CAD build for the part. Positions are in the model's coordinates, mm. Give positions to 0.01 mm unless a question says otherwise; leave off trailing zeros. Write each loop counter-clockwise with the first axis right and the second up, starting at its lowest first coordinate (ties: lowest second). Pieces come first, ordered by that corner, then holes. Notation, with made-up numbers: (44, 29) - (66, 29) arc R22 ccw to (66, 54) - close; hole circle Ø11 at (-17, 64). An arc over 180 degrees is marked (long way). Answer as a JSON object with one key per item and string values.
Autodesk Inventor part; units mm, degrees
ref_plane "YZ Plane" through (0, 0, 0) normal (1, 0, 0) x (0, 1, 0)
ref_plane "XZ Plane" through (0, 0, 0) normal (0, 1, 0) x (-1, 0, 0)
ref_plane "XY Plane" through (0, 0, 0) normal (0, 0, 1) x (1, 0, 0)
sketch "Sketch1" plane through (0, 0, 0) normal (0, 0, 1) x (1, 0, 0)
  line L0 (-47.2309, 58.7326) -> (-58.3434, 58.7326)
  line L1 (-69.4559, 84.1326) -> (-69.4559, 69.8451)
  arc A0 (-69.4559, 69.8451) -> (-58.3434, 58.7326) centre (-58.3434, 69.8451) ccw
  line L2 (-69.4559, 69.8451) -> (-69.4559, 86.6091)
  line L3 (-47.2309, 96.8326) -> (-58.3434, 96.8326)
  line L4 (-69.4559, 85.7201) -> (-69.4559, 86.6091)
  arc A1 (-58.3434, 96.8326) -> (-69.4559, 85.7201) centre (-58.3434, 85.7201) ccw
  line L5 (-47.2309, 46.0326) -> (-66.2809, 46.0326)
  line L6 (-98.0309, 77.7826) -> (-98.0309, 77.7826)
  line L7 (-66.2809, 109.5326) -> (-47.2309, 109.5326)
  arc A2 (-66.2809, 109.5326) -> (-98.0309, 77.7826) centre (-66.2809, 77.7826) ccw
  arc A3 (-98.0309, 77.7826) -> (-66.2809, 46.0326) centre (-66.2809, 77.7826) ccw
  circle A4 centre (-47.2309, 103.1826) radius 2.0955
  circle A5 centre (-47.2309, 52.3826) radius 2.0955
  circle A6 centre (-85.3309, 93.5778) radius 2.0828
  circle A7 centre (-85.3309, 61.9874) radius 2.0828
  line L8 (-47.2309, 96.8326) -> (-21.8309, 96.8326)
  line L9 (-15.4809, 103.1826) -> (-15.4809, 103.1826)
  line L10 (-21.8309, 109.5326) -> (-47.2309, 109.5326)
  line L11 (-47.2309, 58.7326) -> (-21.8309, 58.7326)
  line L12 (-15.4809, 52.3826) -> (-15.4809, 52.3826)
  line L13 (-21.8309, 46.0326) -> (-47.2309, 46.0326)
  arc A8 (-15.4809, 52.3826) -> (-21.8309, 58.7326) centre (-21.8309, 52.3826) ccw
  arc A9 (-21.8309, 46.0326) -> (-15.4809, 52.3826) centre (-21.8309, 52.3826) ccw
  arc A10 (-21.8309, 96.8326) -> (-15.4809, 103.1826) centre (-21.8309, 103.1826) ccw
  arc A11 (-15.4809, 103.1826) -> (-21.8309, 109.5326) centre (-21.8309, 103.1826) ccw
  line L14 (-75.7109, 63.3494) -> (-75.7109, 92.2158)
  arc A12 (-76.923, 92.8904) -> (-76.923, 62.6748) centre (-67.5536, 77.7826) ccw
  arc A13 (-75.7109, 92.2158) -> (-76.923, 92.8904) centre (-76.5047, 92.2158) ccw
  arc A14 (-76.923, 62.6748) -> (-75.7109, 63.3494) centre (-76.5047, 63.3494) ccw
  point P0 (-69.4559, 58.7326)
  point P1 (-15.4809, 58.7326)
  point P2 (-75.7109, 93.5778)
  point P3 (-75.7109, 61.9874)
  dimension "d11" = 22.225
  dimension "d12" = 11.1125
  dimension "d13" = 11.1125
  dimension "d14" = 31.75
  dimension "d15" = 31.75
  dimension "d16" = 4.191
  dimension "d17" = 4.191
  dimension "d18" = 4.1656
  dimension "d19" = 4.1656
  dimension "d21" = 6.35
  dimension "d27" = 0.7937
extrude "Extrusion1" add sketch "Sketch1" along normal blind 1.5875 contours L11 A8 A9 L13 L5 A3 A2 L7 L10 A11 A10 L8 L3 A1 L2 L1 A0 L0 | A14 A12 A13 L14
sketch "Sketch2" plane through (-21.8309, 46.0326, 1.5875) normal (0, 0, 1) x (1, 0, 0)
  circle A0 centre (-24.7079, -19.05) radius 2.3114
  arc A1 (-31.0579, -19.05) -> (-18.4424, -20.0828) centre (-24.7079, -19.05) ccw
  line L0 (-31.0579, -19.05) -> (-31.0579, -6.35)
  line L1 (-44.45, 0) -> (0, 0)
  arc A2 (-31.0579, -6.35) -> (-37.4079, 0) centre (-37.4079, -6.35) ccw
  arc A3 (0, 0) -> (0, 12.7) centre (0, 6.35) ccw
  arc A4 (1.2054, 0.1155) -> (-18.4424, -20.0828) centre (5.886, -24.0929) ccw
  circle A5 centre (25.4, 6.35) radius 2.0955
  line L2 (0, 63.5) -> (-44.45, 63.5)
  arc A6 (0, 50.8) -> (0, 63.5) centre (0, 57.15) ccw
  arc A7 (25.4, 0) -> (25.4, 12.7) centre (25.4, 6.35) ccw
  line L3 (0, 12.7) -> (25.4, 12.7)
  line L4 (0, 0) -> (25.4, 0)
  circle A8 centre (25.4, 57.15) radius 2.0955
  arc A9 (25.4, 50.8) -> (25.4, 63.5) centre (25.4, 57.15) ccw
  line L5 (25.4, 50.8) -> (0, 50.8)
  line L6 (0, 63.5) -> (25.4, 63.5)
  arc A10 (0, 50.8) -> (0, 63.5) centre (0, 57.15) ccw
  point P0 (21.8309, -46.0326)
  point P1 (-31.0579, 0)
  point P2 (0.6434, 0)
  dimension "d22" = 4.6228
  dimension "d24" = 6.35
  dimension "d29" = 4.191
  dimension "d31" = 4.191
  dimension "d32" = 12.7
extrude "Extrusion2" add sketch "Sketch2" against normal blind 1.5875
sketch "Sketch5" plane through (3.5691, 103.1826, 0) normal (0, 0, -1) x (-1, 0, 0)
  line L0 (0, 6.35) -> (69.85, 6.35)
  line L1 (12.7, 0) -> (20.6375, 0) construction
  arc A0 (69.85, -57.15) -> (69.85, 6.35) centre (69.85, -25.4) ccw
  line L2 (69.85, 6.35) -> (50.8, 6.35)
  line L3 (0, 6.35) -> (0, 6.35)
  circle A1 centre (15.875, 25.4) radius 1.905
  arc A2 (0, 6.35) -> (0, -6.35) centre (0, 0) ccw
  line L4 (-6.35, 0) -> (-6.35, 26.9875)
  circle A3 centre (0, 25.4) radius 1.905
  line L5 (-3.175, 30.1625) -> (15.875, 30.1625)
  line L6 (20.6375, 19.05) -> (20.6375, 26.9875)
  line L7 (17.4625, 30.1625) -> (15.875, 30.1625)
  arc A4 (20.6375, 26.9875) -> (17.4625, 30.1625) centre (17.4625, 26.9875) ccw
  arc A5 (-3.175, 30.1625) -> (-6.35, 26.9875) centre (-3.175, 26.9875) ccw
  line L8 (33.3375, 6.35) -> (50.8, 6.35)
  arc A6 (20.6375, 19.05) -> (33.3375, 6.35) centre (33.3375, 19.05) ccw
  point P0 (3.5691, -103.1826)
  point P1 (12.7, 30.1625)
  point P2 (12.7, 6.35)
  point P3 (20.6375, 6.35)
  point P4 (33.3375, 6.35)
  dimension "d33" = 30.1625
  dimension "d37" = 3.81
  dimension "d41" = 3.81
  dimension "d42" = 3.175
  dimension "d43" = 12.7
extrude "Extrusion3" add sketch "Sketch5" against normal blind 1.5875
equation "\"BendRadius\" = Thickness"
equation "\"BendReliefWidth\" = Thickness"
equation "\"BendReliefDepth\" = 0.5 * Thickness"
equation "\"CornerReliefSize\" = 4 * Thickness"
equation "\"MinimumRemnant\" = 2 * Thickness"
equation "\"TransitionRadius\" = BendRadius"
equation "\"JacobiRadiusSize\" = BendRadius"
equation "\"GapSize\" = Thickness"
properties part number "gusset" material "Acetal Resin, White"
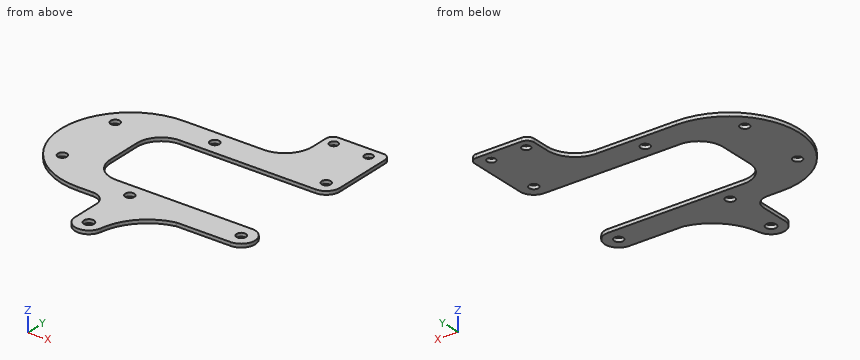
(1) Saw through at C-C, the plane x = -26. Give the cut face in (y, z), and give its area (3 significant figures).
Answer key:
{"outline": "(44.45, 0) - (58.73, 0) - (58.73, 1.59) - (44.45, 1.59) - close; (96.83, 0) - (110.1, 0) - (110.1, 1.59) - (96.83, 1.59) - close", "area": "43.7 mm²"}
(2) Probe L1, parallel to Y at x = -12, z = 0.8; L2, parallel to Y at x = -4, z = 1.45; L3, parallel to Y at x = -47, z = 0.4. List the from-to ranges inside material, lowest first. Write a range as [from, to].
Answer key:
{"L1": "y = [46.03, 58.73], [96.83, 126.7], [130.46, 133.35]", "L2": "y = [46.03, 58.73], [96.83, 133.35]", "L3": "y = [20.65, 24.72], [29.25, 50.3], [54.47, 58.73], [96.83, 101.1], [105.27, 109.53]"}
(3) Saw through at D-D, the plane y = 41. Give the cut face in (x, z).
Answer key:
{"outline": "(-53.03, 0) - (-31.59, 0) - (-31.59, 1.59) - (-53.03, 1.59) - close"}
(4) Flat gauge pins, fed straight in: P1, Ø5, axis at x = 3.57, y = 128.58, coming from the +Z side; P2, Ø4, axis at x = 3.57, y = 103.18, coming from the -Z side; P3, Ø0.5, axis at x = -4, z = 0.5, coming from the -Y side; P4, Ø0.5, axis at y = 126, z = 0.5, coming from the -X side. Where does each tip first touch, or does it go through?
Answer key:
{"P1": "stops at z = 1.59", "P2": "passes through", "P3": "stops at y = 46.03", "P4": "stops at x = -17.07"}
(5) Saw through at A-A, the plane x = -4.5. Give the cut face in (y, z), and give its area (3 significant figures).
Answer key:
{"outline": "(46.03, 0) - (58.73, 0) - (58.73, 1.59) - (46.03, 1.59) - close; (96.83, 0) - (133.35, 0) - (133.35, 1.59) - (96.83, 1.59) - close", "area": "78.1 mm²"}
(6) Saw through at B-B, the plane z = 0.45. State how many separate pieces and enclosed holes the cut face has, and give its area (3 significant figures).
Answer key:
{"separate pieces": "1", "enclosed holes": "9", "area": "4,400 mm²"}
